Answer from the drawing. Dimensions are ordinates in mm from the lowest x, y and z of the part. A direction names the side the tool comes from. Give positions to 0.01 mm unless a question says otherwise; leave off trailing zeros. Loops run counter-clockwise (first coordinate to the right, second up) from the corner with the lowest first, then second, coordinate; pieces in that order, holes last. Notation, with made-up numbers: (31, 30.5) - (69, 30.5) arc R26 cw to (69, 49.5) - close; hole circle Ø10 at (0, 6.5). An arc over 180 degrees is marked (long way). Put each result on its own line as item: value. Start each with the question number.
1. Consider L1, parallel to Y at x = 5.5, z = 5; L2, parallel to Y at x = 6.5, z = 5; L3, parallel to Z at x = 6.75, y = 3. Determine where each line is inside the solid, lowest interval first. Write a range as from..to.
2. For the marked faces 1 and 2, determine the directions among +Z, -Z, +X, -X, +Y, -Y from which every point of the face is accessible in a straight line to the end or side of a thin tool.
3. For a pull along X with two mould halves and no side action, classify the marked faces 3, 4 and 5 as released by +X, released by -X, zero draft, split by the parting line, or undercut.
4. Given pin 1 Ø5 at (y, z) = (9, 12) entering from -X; pin 2 Ø1.5 at (y, z) = (1, 14.5) entering from +X; pin 3 Ø2 at (x, z) = (8.5, 3.5) entering from -Y, each flat-ended and moving along its own axis, determine where each tip first touches the part or whether it passes through.
5. A cutting plane is placed at D-D, the plane z = 15. Determine the outline of the cut face in (x, y), plus the area to 3 significant figures.
6. A cutting plane is placed at A-A, the plane y = 5.5. Determine the outline of the cut face in (x, z).
7. A cutting plane is placed at C-C, the plane z = 1.5. Determine the outline of the cut face in (x, y), plus the area to 3 significant figures.
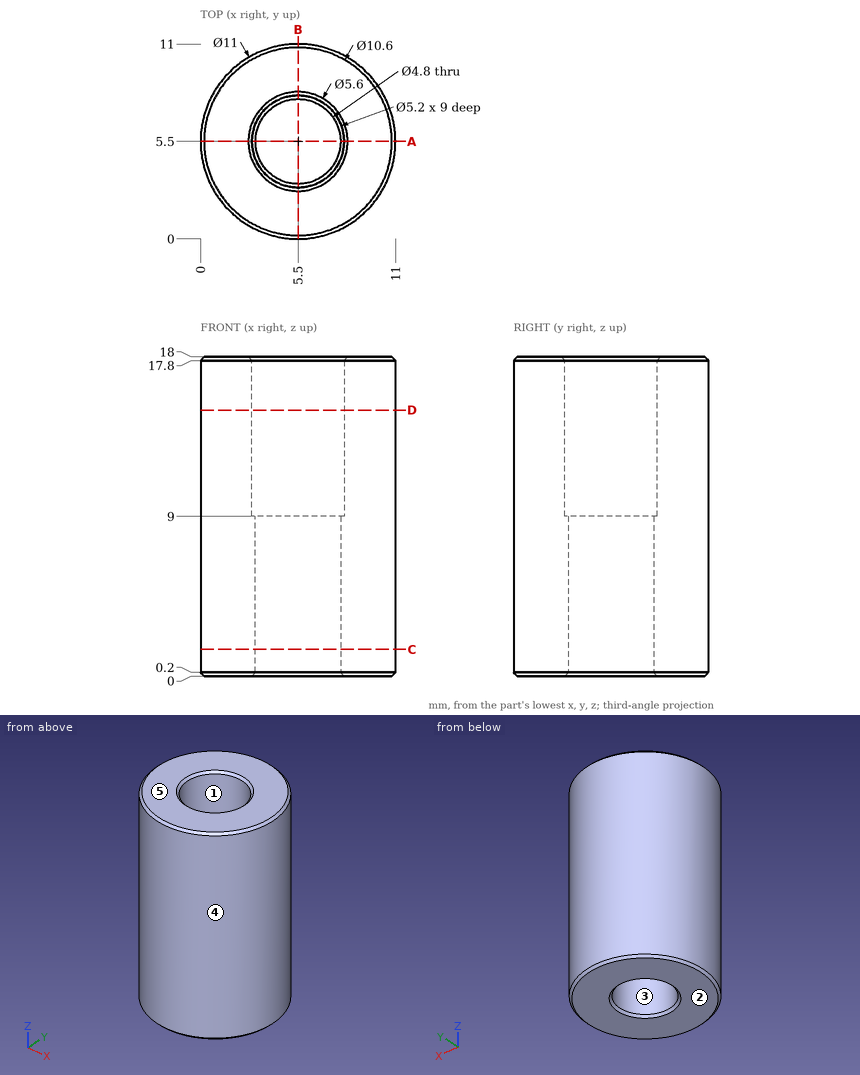
Return value:
1. L1: y = 0..3.1, 7.9..11
1. L2: y = 0.09..3.32, 7.68..10.91
1. L3: z = 0..18
2. face 1: +Z
2. face 2: -Z, +X, -X, +Y, -Y
3. face 3: undercut
3. face 4: split by the parting line
3. face 5: zero draft
4. pin 1: stops at x = 0.09
4. pin 2: stops at x = 9.52
4. pin 3: stops at y = 0.38
5. outline: circle Ø11 at (5.5, 5.5); hole circle Ø5.2 at (5.5, 5.5)
5. area: 73.8 mm2
6. outline: (0, 0.2) - (0.2, 0) - (2.9, 0) - (3.1, 0.2) - (3.1, 9) - (2.9, 9) - (2.9, 17.8) - (2.7, 18) - (0.2, 18) - (0, 17.8) - close; (7.9, 0.2) - (8.1, 0) - (10.8, 0) - (11, 0.2) - (11, 17.8) - (10.8, 18) - (8.3, 18) - (8.1, 17.8) - (8.1, 9) - (7.9, 9) - close
7. outline: circle Ø11 at (5.5, 5.5); hole circle Ø4.8 at (5.5, 5.5)
7. area: 76.9 mm2
